```python
from build123d import *

# Parameters (mm, degrees)
BOSS_EXTRUDE1_DEPTH = 3
SKETCH3_R           = 1.8
CUT_EXTRUDE1_DEPTH  = 3
SKETCH4_W           = 14
SKETCH4_H           = 12
BOSS_EXTRUDE2_DEPTH = 3
BOSS_EXTRUDE3_DEPTH = 14
SKETCH6_W           = 4
SKETCH6_H           = 7
CUT_EXTRUDE2_DEPTH  = 3
FILLET1_R           = 2
FILLET2_R           = 5
FILLET3_R           = 5
FILLET4_R           = 5
SKETCH7_R           = 19
CUT_EXTRUDE3_DEPTH  = 3
FILLET5_R           = 5
FILLET7_R           = 2


with BuildPart() as part:
    # Sketch2 → Boss-Extrude1 (new body)
    with BuildSketch(Plane(origin=(0, 0, 0), x_dir=(1, 0, 0), z_dir=(0, 1, 0))):
        Polygon((0, 10), (13, 20), (27, 20), (40, 10), (40, 0), (0, 0), align=None)
    extrude(amount=BOSS_EXTRUDE1_DEPTH)

    # Sketch3 → Cut-Extrude1 (cut)
    with BuildSketch(Plane(origin=(0, 3, 0), x_dir=(1, 0, 0), z_dir=(0, 1, 0))):
        with Locations(Location((5, 5, 0), (0, 0, 270))):
            Circle(SKETCH3_R)
        with Locations(Location((35, 5, 0), (0, 0, 270))):
            Circle(SKETCH3_R)
    extrude(amount=-CUT_EXTRUDE1_DEPTH, mode=Mode.SUBTRACT)



with BuildPart() as body_2:
    # Sketch4 → Boss-Extrude2 (new body)
    with BuildSketch(Plane(origin=(0, -7.910254038, -13.700961894), x_dir=(-1, 0, 0), z_dir=(0, -0.5000000000000041, -0.8660254037844364))):
        with Locations((-20, 18.598076211)):
            Rectangle(SKETCH4_W, SKETCH4_H)
    extrude(amount=BOSS_EXTRUDE2_DEPTH)


with BuildPart() as part_1:
    add(part.part)

    add(body_2.part)  # Boss-Extrude3 merges body 2
    # Sketch5 → Boss-Extrude3 (add)
    with BuildSketch(Plane.ZY.offset(-13)):
        Polygon((-22.598076211, 1.5), (-20, 0), (-20, 3), align=None)
    extrude(amount=-BOSS_EXTRUDE3_DEPTH)

    # Sketch6 → Cut-Extrude2 (cut)
    with BuildSketch(Plane(origin=(0, -7.910254038, -13.700961894), x_dir=(1, 0, 0), z_dir=(0, 0.5000000000000042, 0.8660254037844363))):
        with Locations((20, 18.098076211)):
            Rectangle(SKETCH6_W, SKETCH6_H)
    extrude(amount=-CUT_EXTRUDE2_DEPTH, mode=Mode.SUBTRACT)

    # Fillet1
    fillet1_edges = [part_1.edges().sort_by_distance(p)[0] for p in [
        (22, 3.982050808, -22.299038106),
        (18, 3.982050808, -22.299038106),
        (18, 10.044228634, -25.799038106),
        (22, 10.044228634, -25.799038106),
    ]]
    fillet(fillet1_edges, radius=FILLET1_R - 0.0001)  # a hair under: the kernel refuses the full size

    # Fillet2
    fillet2_edges = [part_1.edges().sort_by_distance(p)[0] for p in [
        (13, 12.642304845, -27.299038106),
        (27, 12.642304845, -27.299038106),
    ]]
    fillet(fillet2_edges, radius=FILLET2_R)

    # Fillet3
    fillet3_edges = [part_1.edges().sort_by_distance(p)[0] for p in [
        (0, 1.5, -10),
        (40, 1.5, -10),
        (40, 1.5, 0),
        (0, 1.5, 0),
    ]]
    fillet(fillet3_edges, radius=FILLET3_R)

    # Fillet4
    fillet4_edges = [part_1.edges().sort_by_distance(p)[0] for p in [
        (20, 1.5, -22.598076211),
    ]]
    fillet(fillet4_edges, radius=FILLET4_R)

    # Sketch7 → Cut-Extrude3 (cut)
    with BuildSketch(Plane(origin=(0, 3, 0), x_dir=(1, 0, 0), z_dir=(0, 1, 0))):
        with Locations((20, -14)):
            Circle(SKETCH7_R)
    extrude(amount=-CUT_EXTRUDE3_DEPTH, mode=Mode.SUBTRACT)

    # Fillet5
    fillet5_edges = [part_1.edges().sort_by_distance(p)[0] for p in [
        (7.154767421, 1.5, 0),
        (32.845232579, 1.5, 0),
    ]]
    fillet(fillet5_edges, radius=FILLET5_R)

    # Fillet7
    fillet7_edges = [part_1.edges().sort_by_distance(p)[0] for p in [
        (20, 3, -20),
    ]]
    fillet(fillet7_edges, radius=FILLET7_R)


solid = part_1.part
```
Can you work these out from the model? Positions are in its coordinate system, mm. A direction names the side the tool comes from. Coordinates: 2 decimals unless noted, no trailing zeros. Loops run counter-clockwise (first coordinate to the right, second up) from the corner with the lowest first, then second, coordinate; pieces in that order, holes last.
1) Which directions (+Z, -Z, +X, -X, +Y, -Y) give clear straight access to the entire face, cutting with the end or side of a thin tool? Please do faces 1 (the cylindrical face through (25.57, 11.33, -26.57)), 2 (the flat face through (27, 5, -22)), 3 (the flat face through (20, 3, -10)), 4 (the flat face through (13, 5, -22)), 5 (the flat face through (22, 7, -24)).
2) I need wall thicknesses on probe 1 along Y at (x, z) = (11.5, -15.5); probe 2 along X at (y, z) = (1, -2.5); probe 3 along X at (y, z) = (2, -8.25). Which ranges of each line are inside material? Lowest first, please.
3) Thinking about a two-plate mould opening in Z: for faces 6 (the cylindrical face through (33.027, 1.521, -0.275)), 7 (the cylindrical face through (36.785, 1.521, -5.234)), 8 (the cylindrical face through (0.53, 1.52, -9.78)), which applies, pulls with the +Z half, pulls with the -Z half, needs draft (parallel to the pull), parting line crosses it, or undercut?
4) Imagine slicing it at B-B on x = 31. List the corners of the cut face in (y, z) for me.
5) Imagine slicing it at A-A on x = 17. List the corners of the cut face in (y, z) for me.
6) For pin 1 (6 mm diameter, centred on x = 35, z = -5, fed in from +Y); pin 2 (5 mm diameter, centred on y = 6, z = -22, fed in from -X); pin 3 (3 mm diameter, centred on y = 2.5, z = -15.5, fed in from +X), each with a flat end and sliding along its axis, tell me the tip position at first contact or that it passes through.
Completed:
1. face 1: -Z, +X, +Y
1. face 2: -Z, +X, +Y, -Y
1. face 3: +Z, +X, -X, +Y
1. face 4: -Z, -X, +Y, -Y
1. face 5: none
2. probe 1: y = 0 to 3
2. probe 2: x = 0.67 to 10.58, 29.42 to 39.33
2. probe 3: x = 0.05 to 39.95
3. face 6: pulls with the +Z half
3. face 7: undercut
3. face 8: pulls with the -Z half
4. outline: (0, -16.92) - (3, -16.92) - (3, -1.49) - (0, -1.49) - close
5. outline: (0, -20) - (0.83, -21.44) arc R5 ccw to (2.66, -23.27) - (11.8, -28.55) - (13.3, -25.95) - (4, -20.58) arc R2 cw to (3, -18.85) - (3, -4.76) - (0, -4.76) - close
6. pin 1: stops at y = 3
6. pin 2: stops at x = 13
6. pin 3: stops at x = 34.8
